from build123d import *

# Parameters (mm, degrees)
MODEL_R           = 1.4
MODEL_R_2         = 1
BRIDA_BASE1_DEPTH = 1


# Sheet-metal steps are written as plain solids
with BuildPart() as part:
    # Model → Brida base1 (new body)
    with BuildSketch(Plane.XY):
        with BuildLine():
            Line((43.871435578, 46.428949543), (43.688273589, 46.731359657))
            ThreePointArc((43.688273589, 46.731359657), (43.081772243, 47.181843562), (42.333236398, 47.079502368))
            add(Edge.make_bspline(
                [(42.333236398, 47.079502368), (40.764422927, 46.174489073), (35.816548406, 41.900747821), (35.272083644, 35.001949339), (38.359716274, 29.485408266)],
                knots=[0.004002738, 0.004002738, 0.004002738, 0.004002738, 0.255811026, 0.955465838, 0.955465838, 0.955465838, 0.955465838], degree=3))
            ThreePointArc((38.359716274, 29.485408266), (38.416879113, 29.394992141), (38.483372908, 29.311199296))
            Line((38.483372908, 29.311199296), (42.332361737, 24.960661438))
            ThreePointArc((42.332361737, 24.960661438), (42.561250074, 24.507363364), (42.537981803, 24.000088683))
            Line((42.537981803, 24.000088683), (42.240856149, 23.048171958))
            ThreePointArc((42.240856149, 23.048171958), (42.212695742, 22.935208537), (42.197855138, 22.819737764))
            Line((42.197855138, 22.819737764), (40.2059904, -5.7615616))
            Line((40.2059904, -5.7615616), (40.2059904, -15.7615616))
            ThreePointArc((40.2059904, -15.7615616), (45.2059904, -20.7615616), (50.2059904, -15.7615616))
            Line((50.2059904, -15.7615616), (50.2059904, -5.7615616))
            Line((50.2059904, -5.7615616), (48.214125662, 22.819737764))
            ThreePointArc((48.214125662, 22.819737764), (48.199285058, 22.935208537), (48.171124651, 23.048171958))
            Line((48.171124651, 23.048171958), (47.873069238, 24.0030674))
            ThreePointArc((47.873069238, 24.0030674), (47.849307461, 24.508023196), (48.075555852, 24.960081428))
            Line((48.075555852, 24.960081428), (51.860338986, 29.27914154))
            ThreePointArc((51.860338986, 29.27914154), (51.94992334, 29.398217661), (52.020818692, 29.529283781))
            add(Edge.make_bspline(
                [(52.020818692, 29.529283781), (53.24372236, 32.258428286), (54.100570293, 37.543385576), (51.577752865, 42.166423069), (49.399716108, 44.353895199)],
                knots=[0.073238818, 0.073238818, 0.073238818, 0.073238818, 0.521565521, 0.992417875, 0.992417875, 0.992417875, 0.992417875], degree=3))
            Line((49.399716108, 44.353895199), (48.603017078, 45.015390082))
            add(Edge.make_bspline(
                [(48.603017078, 45.015390082), (48.417036758, 45.204787232), (48.174708276, 45.242911079), (47.876031632, 45.129761621)],
                knots=[0, 0, 0, 0, 1, 1, 1, 1], degree=3))
            ThreePointArc((47.876031632, 45.129761621), (47.364904102, 44.467541566), (47.535799978, 43.648651249))
            add(Edge.make_bspline(
                [(47.535799978, 43.648651249), (49.116486798, 41.620539936), (49.633988071, 39.732404237), (48.968154199, 37.939006155)],
                knots=[0, 0, 0, 0, 0.676846712, 0.676846712, 0.676846712, 0.676846712], degree=3))
            add(Edge.make_bspline(
                [(48.968154199, 37.939006155), (48.407530031, 36.24951926), (45.517280844, 35.959596441), (42.879215477, 35.735494746), (42.407543293, 38.017493531)],
                knots=[0, 0, 0, 0, 0.520046034, 1, 1, 1, 1], degree=3))
            add(Edge.make_bspline(
                [(42.407543293, 38.017493531), (42.322809158, 38.308098707), (41.773176484, 40.694157088), (42.398123884, 43.150787581), (43.851661443, 45.361505885)],
                knots=[0.047028419, 0.047028419, 0.047028419, 0.047028419, 0.13151503, 0.738210784, 0.738210784, 0.738210784, 0.738210784], degree=3))
            ThreePointArc((43.851661443, 45.361505885), (44.015919722, 45.892368025), (43.871435578, 46.428949543))
        make_face()
        with Locations((45.2059904, -15.7615616)):
            Circle(MODEL_R, mode=Mode.SUBTRACT)
        with Locations((45.2059904, -3.2615616)):
            Circle(MODEL_R_2, mode=Mode.SUBTRACT)
    extrude(amount=-BRIDA_BASE1_DEPTH)


solid = part.part
Input: part model. Units: mm. Frame: model coordinates. A direction names the side the tool comes from. Coordinates: 2 decimals unless noted, no trailing zeros. Order: outer loops, then holes, each group sorted by start corner. A loop starts at its lowest first (then second) coordinate and runs counter-clockwise, first axis right, second up.
1. Cut plane B-B, the plane y = -9. Return loops of the section in (x, z).
Checked values:
outline: (40.21, -1) - (50.21, -1) - (50.21, 0) - (40.21, 0) - close
2. Cut plane C-C, the plane y = 28. Return loops of the section in (x, z), plus the area to 3 significant figures.
Checked values:
outline: (39.64, -1) - (50.74, -1) - (50.74, 0) - (39.64, 0) - close
area: 11.1 mm2
3. Draft query along Y for faces 4 (the flat face through (45, 14, -1)), 5 (the flat face through (40.38, 27.17, -0.49)), 6 (the cylindrical face through (45.1, -20.76, -0.49)). Return one class per face: +Y half, -Y half, draft (parallel to the pull), parting line (faces both ways), or undercut.
Checked values:
face 4: draft
face 5: undercut
face 6: -Y half
4. Access query for faces 1 (the flat face through (41.216, 8.729, -0.493)), 2 (the flat face through (49.224, 8.329, -0.493)), 3 (the cylindrical face through (44.207, -3.218, -0.493)). Directions: +Z, -Z, +X, -X, +Y, -Y. A direction counts if a zero-diameter tool reaches every point of the face in a straight line with its end or side. Return the directions, or none.
Checked values:
face 1: +Z, -Z, -X
face 2: +Z, -Z, +X
face 3: +Z, -Z
5. Cut plane A-A, the plane z = -0.75. Count the separate pieces of the cut face and the enclosed holes in it, plus the area to 3 significant figures.
Checked values:
separate pieces: 1
enclosed holes: 2
area: 604 mm2
6. Ray query, line 1 along Y through (x, z) = (43, -0.75); line 2 along X through (y, z) = (38.5, -0.2); line 3 along Y through (x, z) = (43.25, -0.35). Return the intervals inside material, ascending.
Checked values:
line 1: y = -20.25 to 36.58, 43.86 to 47.2
line 2: x = 36.3 to 42.28, 49.14 to 53
line 3: y = -20.36 to 36.32, 44.35 to 47.12
